Check sheet for the modelled part. Datum: model origin and axes. Units: mm. A direction names the side the tool comes from. Round coordinates to 2 decimals unless told otherwise and drop trailing zeros. Write each loop counter-clockwise with the first axis right and the second up, starting at its lowest first coordinate (ties: lowest second). Pieces come first, ordered by that corner, then holes.
Item 1: Tool access check on faces 1 (the flat face through (25, 82.55, -541)), 2 (the flat face through (26, 79.375, -541)). Record the directions out of +Z, -Z, +X, -X, +Y, -Y that give a thin tool (end or side, any length) a straight path to the whole face; none if there is none.
Item 2: Cross-section at B-B on y = 52. Enter the section's corners in (x, z) (3 decimals).
Item 3: Material ranges on line 1 (Z direction, x = -1, y = 63); line 2 (Y direction, x = 4, z = -891.5) (3 decimals); line 3 (X direction, y = 3.5, z = -876) (3 decimals), recorded low to high.
Item 4: Cross-section at A-A on z = -157.5. Enter the section's corners in (x, y) (3 decimals).
Item 5: Go/stop test with flat-tipped pins: pin 1 Ø8 at (y, z) = (63.5, -28.575) entering from +X; pin 2 Ø3.5 at (y, z) = (81.5, -206.5) entering from +X (3 decimals); pin 3 Ø3.5 at (x, y) = (39, 81) entering from -Z. Record where each tip stops, or that it passes through.
from build123d import *

# Parameters (mm, degrees)
SKETCH1_W                    = 1066.8
SKETCH1_H                    = 82.55
BASE_FLANGE1_DEPTH           = 3.175
EDGE_FLANGE1_STRIP_W         = 19.05
EDGE_FLANGE1_STRIP_H         = 3.175
EDGE_FLANGE1_STRIP_CUT_DEPTH = 1066.8
EDGE_FLANGE1_DEPTH           = 1066.8
SKETCH9_R                    = 2.45745
CUT_EXTRUDE1_DEPTH           = 1072.688316688
SKETCH10_R                   = 4.3688
CUT_EXTRUDE2_DEPTH           = 3.175
FILLET1_R                    = 6.35


# Sheet-metal steps are written as plain solids
with BuildPart() as part:
    # Sketch1 → Base-Flange1 (new body)
    with BuildSketch(Plane(origin=(0, 0, 0), x_dir=(0, 0, -1), z_dir=(1, 0, 0))):
        with Locations((533.4, 41.275)):
            Rectangle(SKETCH1_W, SKETCH1_H)
    extrude(amount=-BASE_FLANGE1_DEPTH)

    # Edge-Flange1 strip (across the edge) → Edge-Flange1 strip cut (cut)
    with BuildSketch(Plane(origin=(0, 82.55, -1066.8), x_dir=(0, -1, 0), z_dir=(0, 0, 1))):
        with Locations((-3.175, -1.5875)):
            Rectangle(EDGE_FLANGE1_STRIP_W, EDGE_FLANGE1_STRIP_H)
    extrude(amount=EDGE_FLANGE1_STRIP_CUT_DEPTH, mode=Mode.SUBTRACT)

    # Edge-Flange1 section (across the edge) → Edge-Flange1 (add)
    with BuildSketch(Plane(origin=(0, 82.55, -1066.8), x_dir=(0, -1, 0), z_dir=(0, 0, 1))):
        with BuildLine():
            Line((0, 3.175), (0, 60.325))
            Line((0, 60.325), (3.175, 60.325))
            Line((3.175, 60.325), (3.175, 3.175))
            ThreePointArc((3.175, 3.175), (4.10493597, 0.92993597), (6.35, 0))
            Line((6.35, 0), (6.35, -3.175))
            ThreePointArc((6.35, -3.175), (1.859871939, -1.315128061), (0, 3.175))
        make_face()
    extrude(amount=EDGE_FLANGE1_DEPTH)

    # Sketch9 → Cut-Extrude1 (cut, through all)
    with BuildSketch(Plane(origin=(0, 0, 0), x_dir=(0, 0, -1), z_dir=(1, 0, 0))):
        with Locations((28.575, 63.5)):
            Circle(SKETCH9_R)
        with Locations((200.025, 63.5)):
            Circle(SKETCH9_R)
        with Locations((28.575, 15.875)):
            Circle(SKETCH9_R)
        with Locations((200.025, 15.875)):
            Circle(SKETCH9_R)
        with Locations(Location((866.775, 63.5, 0), (0, 0, 180))):
            Circle(SKETCH9_R)
        with Locations(Location((866.775, 15.875, 0), (0, 0, 180))):
            Circle(SKETCH9_R)
        with Locations(Location((1038.225, 15.875, 0), (0, 0, 180))):
            Circle(SKETCH9_R)
        with Locations(Location((1038.225, 63.5, 0), (0, 0, 180))):
            Circle(SKETCH9_R)
    extrude(amount=-CUT_EXTRUDE1_DEPTH, mode=Mode.SUBTRACT)

    # Sketch10 → Cut-Extrude2 (cut)
    with BuildSketch(Plane(origin=(0, 82.55, 0), x_dir=(1, 0, 0), z_dir=(0, 1, 0))):
        with Locations(Location((41.275, 650.875, 0), (0, 0, 180))):
            Circle(SKETCH10_R)
        with Locations(Location((41.275, 415.925, 0), (0, 0, 180))):
            Circle(SKETCH10_R)
        Polygon((15.875, 1066.8), (79.375, 1066.8), (79.375, 0), (15.875, 0), (15.875, 400.05), (60.325, 400.05), (60.325, 666.75), (15.875, 666.75), align=None)
    extrude(amount=-CUT_EXTRUDE2_DEPTH, mode=Mode.SUBTRACT)

    # Fillet1
    fillet1_edges = [part.edges().sort_by_distance(p)[0] for p in [
        (15.875, 80.9625, -1066.8),
        (15.875, 80.9625, -666.75),
        (15.875, 80.9625, 0),
        (15.875, 80.9625, -400.05),
        (60.325, 80.9625, -400.05),
        (60.325, 80.9625, -666.75),
        (-1.5875, 0, 0),
        (-1.5875, 0, -1066.8),
    ]]
    fillet(fillet1_edges, radius=FILLET1_R)


solid = part.part
Response values:
1. face 1: +Z, -Z, +X, -X, +Y
1. face 2: +Z, -Z, +X, -Y
2. outline: (-3.175, -1066.8) - (0, -1066.8) - (0, 0) - (-3.175, 0) - close
3. line 1: z = -1066.8 to -1040.63, -1035.82 to -869.18, -864.37 to -202.43, -197.62 to -30.98, -26.17 to 0
3. line 2: y = 79.375 to 82.55
3. line 3: x = -3.175 to 0
4. outline: (-3.175, 0) - (0, 0) - (0, 76.2) arc R3.175 cw to (3.175, 79.375) - (15.875, 79.375) - (15.875, 82.55) - (3.175, 82.55) arc R6.35 ccw to (-3.175, 76.2) - close
5. pin 1: stops at x = 0
5. pin 2: stops at x = 15.875
5. pin 3: stops at z = -666.75
